```python
from build123d import *

# Parameters (mm, degrees)
SKETCH1_W               = 38
SKETCH1_H               = 60
BOSS_EXTRUDE1_DEPTH     = 9
CUT_EXTRUDE1_DEPTH      = 1
CUT_EXTRUDE1_DEPTH_BACK = 18
SKETCH5_R               = 3
CUT_EXTRUDE2_DEPTH      = 38
CHAMFER1_SIZE           = 2


with BuildPart() as part:
    # Sketch1 → Boss-Extrude1 (new body, symmetric)
    with BuildSketch(Plane.XY):
        with Locations((0, 30)):
            Rectangle(SKETCH1_W, SKETCH1_H)
    extrude(amount=BOSS_EXTRUDE1_DEPTH, both=True)

    # Sketch2 → Cut-Extrude1 (cut, two sides)
    with BuildSketch(Plane.XY.offset(9)) as cut_extrude1_sk:
        Polygon((-15.5, 2.5), (-15.5, 0), (15.5, 0), (15.5, 2.5), (13, 2.5), (13, 5), (10.5, 5), (10.5, 7.5), (8, 7.5), (8, 10), (5.5, 10), (5.5, 12.5), (3, 12.5), (3, 15), (-3, 15), (-3, 12.5), (-5.5, 12.5), (-5.5, 10), (-8, 10), (-8, 7.5), (-10.5, 7.5), (-10.5, 5), (-13, 5), (-13, 2.5), align=None)
    extrude(amount=CUT_EXTRUDE1_DEPTH, mode=Mode.SUBTRACT)
    extrude(cut_extrude1_sk.sketch, amount=-CUT_EXTRUDE1_DEPTH_BACK, mode=Mode.SUBTRACT)

    # Sketch4 → Cut-Revolve1 (revolve, cut)
    with BuildSketch(Plane.XY):
        Polygon((-6, 60), (-6, 40), (0, 36.535898385), (0, 60), align=None)
    revolve(axis=Axis((0, 73.07179677, 0), (0, -1, 0)), mode=Mode.SUBTRACT)

    # Sketch5 → Cut-Extrude2 (cut)
    with BuildSketch(Plane(origin=(19, 0, 0), x_dir=(0, 0, -1), z_dir=(1, 0, 0))):
        with Locations((0, 53)):
            Circle(SKETCH5_R)
    extrude(amount=-CUT_EXTRUDE2_DEPTH, mode=Mode.SUBTRACT)

    # Chamfer1
    chamfer1_edges = [part.edges().sort_by_distance(p)[0] for p in [
        (0, 60, 9),
        (0, 60, -9),
        (-19, 60, 0),
        (19, 60, 0),
    ]]
    chamfer(chamfer1_edges, length=CHAMFER1_SIZE)


solid = part.part
```
Can you work these out from the model? Positions are in its coordinate system, mm. A direction names the side the tool comes from. Give positions to 0.01 mm unless a question says otherwise; leave off trailing zeros. Write each loop counter-clockwise with the first axis right and the second up, starting at its lowest first coordinate (ties: lowest second). Pieces come first, ordered by that corner, then holes. Notation, with made-up numbers: (-21, 1) -> (-15, 1) arc R19 cw to (-15, 8) -> close; hole circle Ø9 at (-13.75, 43.25). An arc over 180 degrees is marked (long way). One line per item, written item: value.
Q1. For P1, Ø6, axis at x = -3, z = 1.5, coming from the -Y side; P2, Ø5, axis at x = -1, z = 1.5, coming from the -Y side; P3, Ø1.5, axis at x = -14, z = -1, coming from the -Y side, each with a flat end and sliding along its axis, tell me the tip position at first contact or that it passes through.
Results found:
P1: stops at y = 10
P2: stops at y = 12.5
P3: stops at y = 2.5
Q2. Imagine slicing it at A-A on y = 53. Please give me the cut outline in (x, z), and give its area (3 significant figures).
Results found:
outline: (-19, -9) -> (19, -9) -> (19, -3) -> (5.2, -3) arc R6 cw to (-5.2, -3) -> (-19, -3) -> close; (-19, 3) -> (-5.2, 3) arc R6 cw to (5.2, 3) -> (19, 3) -> (19, 9) -> (-19, 9) -> close
area: 412 mm^2
Q3. Please list where these lines run through material, in increasing order: line 1 (Z direction, x = 10.5, y = 53); line 2 (X direction, y = 11.5, z = 7.5); line 3 (Z direction, x = 0, y = 54). Write a range as [from, to].
Results found:
line 1: z = [-9, -3], [3, 9]
line 2: x = [-19, -5.5], [5.5, 19]
line 3: z = [-9, -6], [6, 9]
Q4. Imagine slicing it at C-C on y = 44.5. Please give me the cut outline in (x, z).
Results found:
outline: (-19, -9) -> (19, -9) -> (19, 9) -> (-19, 9) -> close; hole circle Ø12 at (0, 0)
Q5. We'd pull the mould along X, two halves only. Please class faces 3 (the face through (0, 36, -9)), 4 (the face through (-7, 10, 0)), 5 (the face through (-19, 29, 0)): +X half, -X half, draft (parallel to the pull), parting line (faces both ways), or undercut.
Results found:
face 3: draft
face 4: undercut
face 5: -X half
Q6. Imagine slicing it at B-B on x = 9.5. Please give me the cut outline in (y, z), and give its area (3 significant figures).
Results found:
outline: (7.5, -9) -> (58, -9) -> (60, -7) -> (60, 7) -> (58, 9) -> (7.5, 9) -> close; hole circle Ø6 at (53, 0)
area: 913 mm^2
Q7. Imagine slicing it at D-D on z = 2.25. Give the number of separate pieces and of enclosed holes in the cut face, and give its area (3 significant figures).
Results found:
separate pieces: 3
enclosed holes: 0
area: 1,650 mm^2
Q8. Which directions (+Z, -Z, +X, -X, +Y, -Y) give clear straight access to the entire face, cutting with the end or side of a thin tool? Please do faces 1 (the face through (-4, 60, 5)), 2 (the face through (8, 9, 0)).
Results found:
face 1: +Z, -Z, +X, -X, +Y
face 2: +Z, -Z, -Y
